Part model, mm, in its own coordinate system. Give positions to 0.01 mm unless a question says otherwise; leave off trailing zeros. Order: outer loops, then holes, each group sorted by start corner. A loop starts at its lowest first (then second) coordinate and runs counter-clockwise, first axis right, second up. Notation, with made-up numbers: (59, 35) -> (104, 35) arc R20 cw to (104, 57) -> close; hole circle Ø7 at (67.5, 7.25). An arc over 180 degrees is marked (long way). Write item = value, one per line. Start each with the question number.
(1) Probe line 1 along Y through (x, z) = (47, 0.6); line 2 along X through (y, z) = (-55, 2.4); line 3 along X through (y, z) = (62, 3.75). List the from-to ranges inside material, lowest first. Write a range as from..to.
(2) Saw through at D-D, the plane z = 0.8. State how many separate pieces and enclosed holes the cut face has, then the cut area to 3 significant figures.
(3) Saw through at A-A, the plane y = 0. List the corners of the cut face in (x, z).
(4) Flat gauge pins, fed straight in: pin 1 (4 mm diameter, centred on x = -19.8, y = 19.8, fed in from +Z); pin 2 (1.5 mm diameter, centred on x = 47, z = 1.5, fed in from -Y). Where does each tip first touch, or does it go through?
(5) Saw through at C-C, the plane y = -48.5. List the corners of the cut face in (x, z).
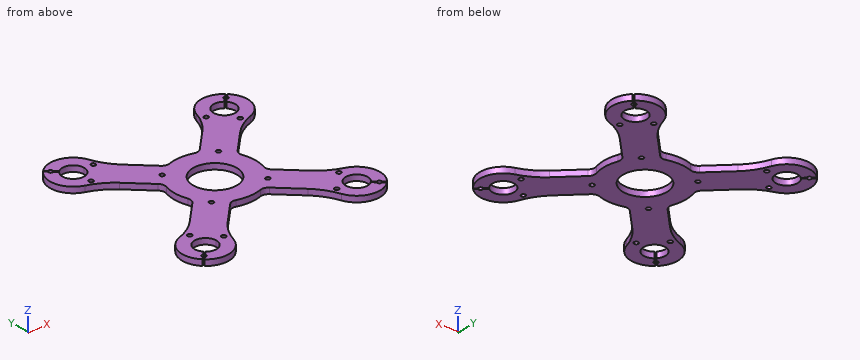
from build123d import *

# Parameters (mm, degrees)
SKETCH1_R           = 1.5
SKETCH1_R_2         = 7.5
SKETCH1_R_3         = 15
BOSS_EXTRUDE1_DEPTH = 4
CUT_EXTRUDE2_DEPTH  = 98.709326831
FILLET3_R           = 40
FILLET4_R           = 5


with BuildPart() as part:
    # Sketch1 → Boss-Extrude1 (new body)
    with BuildSketch(Plane.XY):
        with BuildLine():
            Line((37.130179911, 51.272315535), (11.422174197, 25.564309821))
            ThreePointArc((11.422174197, 25.564309821), (0, 28), (-11.422174197, 25.564309821))
            Line((-11.422174197, 25.564309821), (-37.130179911, 51.272315535))
            ThreePointArc((-37.130179911, 51.272315535), (-64.346717088, 64.346717088), (-51.272315535, 37.130179911))
            Line((-51.272315535, 37.130179911), (-25.564309821, 11.422174197))
            ThreePointArc((-25.564309821, 11.422174197), (-28, 0), (-25.564309821, -11.422174197))
            Line((-25.564309821, -11.422174197), (-51.272315535, -37.130179911))
            ThreePointArc((-51.272315535, -37.130179911), (-64.346717088, -64.346717088), (-37.130179911, -51.272315535))
            Line((-37.130179911, -51.272315535), (-11.422174197, -25.564309821))
            ThreePointArc((-11.422174197, -25.564309821), (0, -28), (11.422174197, -25.564309821))
            Line((11.422174197, -25.564309821), (37.130179911, -51.272315535))
            ThreePointArc((37.130179911, -51.272315535), (64.346717088, -64.346717088), (51.272315535, -37.130179911))
            Line((51.272315535, -37.130179911), (25.564309821, -11.422174197))
            ThreePointArc((25.564309821, -11.422174197), (28, 0), (25.564309821, 11.422174197))
            Line((25.564309821, 11.422174197), (51.272315535, 37.130179911))
            ThreePointArc((51.272315535, 37.130179911), (64.346717088, 64.346717088), (37.130179911, 51.272315535))
        make_face()
        with Locations((52.325901808, 39.597979746)):
            Circle(SKETCH1_R, mode=Mode.SUBTRACT)
        with Locations((19.798989873, -19.798989873)):
            Circle(SKETCH1_R, mode=Mode.SUBTRACT)
        with Locations((61.518289963, 61.518289963)):
            Circle(SKETCH1_R, mode=Mode.SUBTRACT)
        with Locations((-19.798989873, -19.798989873)):
            Circle(SKETCH1_R, mode=Mode.SUBTRACT)
        with Locations((19.798989873, 19.798989873)):
            Circle(SKETCH1_R, mode=Mode.SUBTRACT)
        with Locations((-19.798989873, 19.798989873)):
            Circle(SKETCH1_R, mode=Mode.SUBTRACT)
        with Locations((39.597979746, 52.325901808)):
            Circle(SKETCH1_R, mode=Mode.SUBTRACT)
        with Locations((53.033008589, 53.033008589)):
            Circle(SKETCH1_R_2, mode=Mode.SUBTRACT)
        with Locations((53.033008589, -53.033008589)):
            Circle(SKETCH1_R_2, mode=Mode.SUBTRACT)
        with Locations((61.518289963, -61.518289963)):
            Circle(SKETCH1_R, mode=Mode.SUBTRACT)
        with Locations((52.325901808, -39.597979746)):
            Circle(SKETCH1_R, mode=Mode.SUBTRACT)
        with Locations((39.597979746, -52.325901808)):
            Circle(SKETCH1_R, mode=Mode.SUBTRACT)
        with Locations((-53.033008589, -53.033008589)):
            Circle(SKETCH1_R_2, mode=Mode.SUBTRACT)
        with Locations((-61.518289963, -61.518289963)):
            Circle(SKETCH1_R, mode=Mode.SUBTRACT)
        with Locations((-39.597979746, -52.325901808)):
            Circle(SKETCH1_R, mode=Mode.SUBTRACT)
        with Locations((-52.325901808, -39.597979746)):
            Circle(SKETCH1_R, mode=Mode.SUBTRACT)
        with Locations((-53.033008589, 53.033008589)):
            Circle(SKETCH1_R_2, mode=Mode.SUBTRACT)
        with Locations((-61.518289963, 61.518289963)):
            Circle(SKETCH1_R, mode=Mode.SUBTRACT)
        with Locations((-52.325901808, 39.597979746)):
            Circle(SKETCH1_R, mode=Mode.SUBTRACT)
        with Locations((-39.597979746, 52.325901808)):
            Circle(SKETCH1_R, mode=Mode.SUBTRACT)
        Circle(SKETCH1_R_3, mode=Mode.SUBTRACT)
    extrude(amount=BOSS_EXTRUDE1_DEPTH)

    # Sketch3 → Cut-Extrude2 (cut, through all)
    with BuildSketch(Plane.XY.offset(4)):
        Polygon((63.993163697, 64.700270479), (57.970957821, 58.678064602), (58.678064602, 57.970957821), (64.700270479, 63.993163697), align=None)
        Polygon((58.678064602, -57.970957821), (57.970957821, -58.678064602), (63.993163697, -64.700270479), (64.700270479, -63.993163697), align=None)
        Polygon((-57.970957821, -58.678064602), (-58.678064602, -57.970957821), (-64.700270479, -63.993163697), (-63.993163697, -64.700270479), align=None)
        Polygon((-58.678064602, 57.970957821), (-57.970957821, 58.678064602), (-63.993163697, 64.700270479), (-64.700270479, 63.993163697), align=None)
    extrude(amount=-CUT_EXTRUDE2_DEPTH, mode=Mode.SUBTRACT)

    # Fillet3
    fillet3_edges = [part.edges().sort_by_distance(p)[0] for p in [
        (37.130179911, 51.272315535, 2),
        (51.272315535, 37.130179911, 2),
        (51.272315535, -37.130179911, 2),
        (37.130179911, -51.272315535, 2),
        (-37.130179911, -51.272315535, 2),
        (-51.272315535, -37.130179911, 2),
        (-51.272315535, 37.130179911, 2),
        (-37.130179911, 51.272315535, 2),
    ]]
    fillet(fillet3_edges, radius=FILLET3_R)

    # Fillet4
    fillet4_edges = [part.edges().sort_by_distance(p)[0] for p in [
        (11.422174197, 25.564309821, 2),
        (25.564309821, 11.422174197, 2),
        (25.564309821, -11.422174197, 2),
        (11.422174197, -25.564309821, 2),
        (-11.422174197, -25.564309821, 2),
        (-25.564309821, -11.422174197, 2),
        (-25.564309821, 11.422174197, 2),
        (-11.422174197, 25.564309821, 2),
    ]]
    fillet(fillet4_edges, radius=FILLET4_R)


solid = part.part
Results list:
q1.line_1 = -67.85..-57.49, -48.58..-32.17, 32.17..48.58, 57.49..67.85
q1.line_2 = -68.91..-60.27, -45.8..-36.7, 36.7..45.8, 60.27..68.91
q1.line_3 = -66.28..-62.94, -60.1..-39.78, 39.78..60.1, 62.94..66.28
q2.separate_pieces = 1
q2.enclosed_holes = 13
q2.area = 6,860 mm^2
q3.outline = (-28, 0) -> (-15, 0) -> (-15, 4) -> (-28, 4) -> close; (15, 0) -> (28, 0) -> (28, 4) -> (15, 4) -> close
q4.pin_1 = 4
q4.pin_2 = -68.14
q5.outline = (-68.38, 0) -> (-59.01, 0) -> (-59.01, 4) -> (-68.38, 4) -> close; (-47.06, 0) -> (-33.21, 0) -> (-33.21, 4) -> (-47.06, 4) -> close; (33.21, 0) -> (47.06, 0) -> (47.06, 4) -> (33.21, 4) -> close; (59.01, 0) -> (68.38, 0) -> (68.38, 4) -> (59.01, 4) -> close
